CAD build for the part. Positions are in the model's coordinates, mm. A direction names the side the tool comes from. Round coordinates to 2 decimals unless told otherwise and drop trailing zeros. Order: outer loops, then holes, each group sorted by start corner. A loop starts at its lowest first (then second) coordinate and runs counter-clockwise, first axis right, second up. Notation, with made-up numbers: (-22.5, -3.75) -> (-15.5, -3.75) arc R16 cw to (-15.5, 4.25) -> close; hole circle Ø9 at (3.25, -37). An arc over 180 degrees is marked (long way). Return JSON: item names as keys, results as strings. Group by question number.
Q1. Which spindle directions (+Z, -Z, +X, -X, +Y, -Y) get a long thin tool onto all of the face, cutting with end or side? Do faces 1 (the flat face through (-14, 3, 21.25)), 2 (the flat face through (-274, 3, 124)), 3 (the flat face through (-274, 3, 40)). Say none if no direction does.
Q2. Flat gauge pins, fed straight in: pin 1 (1.2 mm diameter, centred on y = 3, z = 22.5, fed in from +X); pin 2 (3 mm diameter, centred on x = -275, y = 3, fed in from -Z); pin 3 (2 mm diameter, centred on y = 3.5, z = 156, fed in from +X). Where does each tip first touch, or does it go through?
Q3. Probe line 1 along X through (y, z) = (5.1, 22); line 2 along X through (y, z) = (4.55, 61). List the from-to ranges inside material, lowest first.
Q4. Cut at A-A (z = 162). Write the cut outline in (x, y), then the cut area to 3 significant figures.
Autodesk Inventor part; units mm, degrees
ref_plane "YZ Plane" through (0, 0, 0) normal (1, 0, 0) x (0, 1, 0)
ref_plane "XZ Plane" through (0, 0, 0) normal (0, 1, 0) x (-1, 0, 0)
ref_plane "XY Plane" through (0, 0, 0) normal (0, 0, 1) x (1, 0, 0)
sketch "Sketch1" plane through (0, 0, 0) normal (0, 1, 0) x (-1, 0, 0)
  line L0 (0, 0) -> (271, 0)
  line L1 (271, 0) -> (271, 176)
  line L2 (271, 176) -> (0, 176)
  line L3 (0, 176) -> (0, 0)
  line L4 (-6, 136) -> (0, 136)
  line L5 (0, 136) -> (0, 124)
  line L6 (0, 124) -> (-6, 124)
  line L7 (-6, 124) -> (-6, 136)
  line L8 (-6, 94) -> (0, 94)
  line L9 (0, 94) -> (0, 82)
  line L10 (0, 82) -> (-6, 82)
  line L11 (-6, 82) -> (-6, 94)
  line L12 (-6, 52) -> (0, 52)
  line L13 (0, 52) -> (0, 40)
  line L14 (0, 40) -> (-6, 40)
  line L15 (-6, 40) -> (-6, 52)
  circle A0 centre (-3, 156) radius 1.25
  circle A1 centre (-3, 20) radius 1.25
  line L16 (-3, 40) -> (-3, 20) construction
  line L17 (135.5, 176) -> (135.5, 0) construction
  line L18 (277, 40) -> (277, 52)
  line L19 (271, 40) -> (277, 40)
  line L20 (271, 52) -> (271, 40)
  line L21 (277, 52) -> (271, 52)
  line L22 (271, 82) -> (277, 82)
  line L23 (277, 94) -> (271, 94)
  line L24 (271, 94) -> (271, 82)
  line L25 (277, 82) -> (277, 94)
  line L26 (271, 124) -> (277, 124)
  line L27 (271, 136) -> (271, 124)
  line L28 (277, 136) -> (271, 136)
  line L29 (277, 124) -> (277, 136)
  point P0 (274, 40)
  dimension "d0" = 271
  dimension "d2" = 6
  dimension "d3" = 12
  dimension "d4" = 30
  dimension "d5" = 30
  dimension "d6" = 2.5
  dimension "d7" = 2.5
  dimension "d8" = 20
  dimension "d9" = 20
  dimension "d10" = 20
  dimension "d13" = 20
extrude "Extrusion1" add sketch "Sketch1" along normal blind 6 contours L3 L2 L1 L0 | L14 L15 L12 L3 | L1 L21 L18 L19 | L10 L11 L8 L3 | L1 L23 L25 L22 | L6 L7 L4 L3 | L1 L28 L29 L26
sketch "Sketch2" plane through (0, 6, 0) normal (0, 1, 0) x (1, 0, 0)
  line L0 (0, -40) -> (0, 0)
  line L1 (0, -18.75) -> (-8, -18.75)
  line L2 (-17, -18.75) -> (-17, -21.25)
  line L3 (-17, -21.25) -> (-10.3, -21.25)
  line L4 (0, -21.25) -> (0, -18.75)
  line L5 (0, 0) -> (-271, 0)
  line L6 (-8, -22.7) -> (-10.3, -22.7)
  line L7 (-10.3, -22.7) -> (-10.3, -21.25)
  line L8 (-10.3, -17.3) -> (-8, -17.3)
  line L9 (-8, -17.3) -> (-8, -18.75)
  line L10 (-8, -21.25) -> (-8, -22.7)
  line L11 (-8, -18.75) -> (-8, -21.25) construction
  line L12 (-10.3, -21.25) -> (-10.3, -18.75) construction
  line L13 (-10.3, -18.75) -> (-10.3, -17.3)
  line L14 (-8, -21.25) -> (0, -21.25)
  line L15 (-10.3, -21.25) -> (-8, -21.25) construction
  line L16 (-8, -18.75) -> (-10.3, -18.75) construction
  line L17 (-10.3, -18.75) -> (-17, -18.75)
  line L18 (0, -154.75) -> (-8, -154.75)
  line L19 (-17, -154.75) -> (-17, -157.25)
  line L20 (-17, -157.25) -> (-10.3, -157.25)
  line L21 (0, -157.25) -> (0, -154.75)
  line L22 (-8, -158.7) -> (-10.3, -158.7)
  line L23 (-10.3, -158.7) -> (-10.3, -157.25)
  line L24 (-10.3, -153.3) -> (-8, -153.3)
  line L25 (-8, -153.3) -> (-8, -154.75)
  line L26 (-8, -157.25) -> (-8, -158.7)
  line L27 (-8, -154.75) -> (-8, -157.25) construction
  line L28 (-10.3, -157.25) -> (-10.3, -154.75) construction
  line L29 (-10.3, -154.75) -> (-10.3, -153.3)
  line L30 (-8, -157.25) -> (0, -157.25)
  line L31 (-10.3, -157.25) -> (-8, -157.25) construction
  line L32 (-8, -154.75) -> (-10.3, -154.75) construction
  line L33 (-10.3, -154.75) -> (-17, -154.75)
  line L34 (0, -176) -> (0, -136)
  line L35 (-271, -176) -> (0, -176)
  dimension "d14" = 17
  dimension "d15" = 2.5
  dimension "d16" = 18.75
  dimension "d19" = 2.3
  dimension "d20" = 5.4
  dimension "d21" = 8
  dimension "d22" = 17
  dimension "d23" = 2.5
  dimension "d24" = 2.3
  dimension "d25" = 5.4
  dimension "d26" = 18.75
extrude "Extrusion2" cut sketch "Sketch2" against normal through all
equation "\"d5\" = d4"
equation "\"d6\" = d7"
equation "\"d9\" = d8"
equation "\"d26\" = d16"
properties part number "pinball-case-back"
Solution:
{
 "1": {"face 1": "+X, +Y, -Y", "face 2": "-X, +Y, -Y", "face 3": "-Z, -X, +Y, -Y"},
 "2": {"pin 1": "stops at x = 0", "pin 2": "stops at z = 40", "pin 3": "stops at x = -17"},
 "3": {"line 1": "x = -271 to -10.3, -8 to 0", "line 2": "x = -271 to 0"},
 "4": {"outline": "(-271, 0) -> (0, 0) -> (0, 6) -> (-271, 6) -> close", "area": "1,630 mm²"}
}
